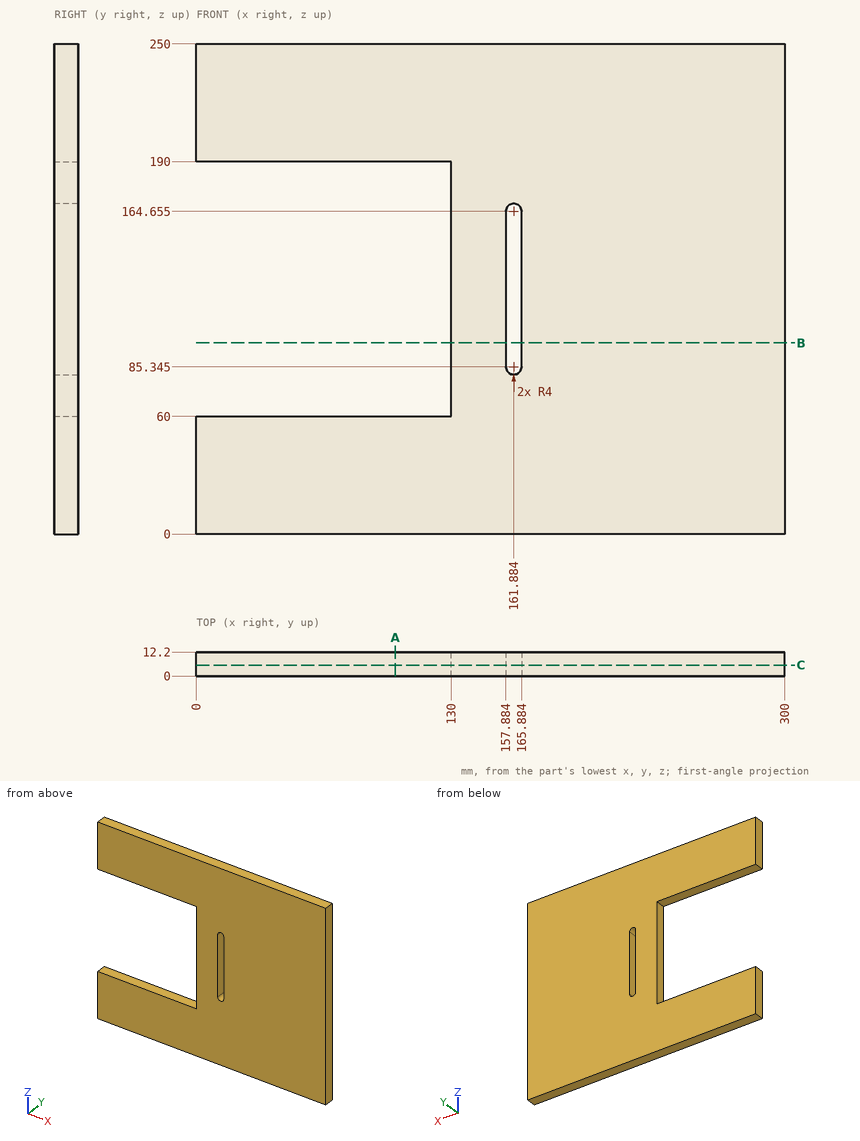
The drawing under review shows one solid part. Ordinate dimensions are in mm from its lowest x, y, z. Coordinates: 2 decimals unless noted, no trailing zeros. Order: outer loops, then holes, each group sorted by start corner. A loop starts at its lowest first (then second) coordinate and runs counter-clockwise, first axis right, second up. Notation, with made-up numbers: (-24, -33) -> (10, -33) arc R34 cw to (10, 6) -> close; hole circle Ø6 at (42.25, 43.25). An arc over 180 degrees is marked (long way). Answer as CSV lines item,"result".
Q1. We need section B-B (z = 97.5). State the section outline as (x, y) points (1 decimal).
Model answer:
outline,"(130, 0) -> (157.9, 0) -> (157.9, 12.2) -> (130, 12.2) -> close; (165.9, 0) -> (300, 0) -> (300, 12.2) -> (165.9, 12.2) -> close"
Q2. Clearance check with flat-ended pins moving along their axes: pin 1 Ø3.5 at (x, y) = (74, 6.5) entering from -Z; pin 2 Ø2 at (y, z) = (4, 82) entering from -X. State where each tip first meets the part, or that it passes through.
Model answer:
pin 1,"stops at z = 0"
pin 2,"stops at x = 130"
Q3. We need section A-A (x = 101.5). State the section outline as (y, z) points, plus the area to 3 significant figures.
Model answer:
outline,"(0, 0) -> (12.2, 0) -> (12.2, 60) -> (0, 60) -> close; (0, 190) -> (12.2, 190) -> (12.2, 250) -> (0, 250) -> close"
area,"1,460 mm2"
Q4. We need section C-C (y = 5.5). State the section outline as (x, z) points (1 decimal), plus the area to 3 significant figures.
Model answer:
outline,"(0, 0) -> (300, 0) -> (300, 250) -> (0, 250) -> (0, 190) -> (130, 190) -> (130, 60) -> (0, 60) -> close; hole (157.9, 85.3) arc R4 ccw to (165.9, 85.3) -> (165.9, 164.7) arc R4 ccw to (157.9, 164.7) -> close"
area,"57,400 mm2"
Q5. Wall thickness on line 1 along X through (y, z) = (3, 120.5) (1 decimal); line 2 along Z through (x, y) = (79, 11.75); line 3 along X through (y, z) = (8.25, 62): over which ranges is each line inside the solid? List them lowest first. Write a range as [from, to].
Model answer:
line 1,"x = [130, 157.9], [165.9, 300]"
line 2,"z = [0, 60], [190, 250]"
line 3,"x = [130, 300]"
